The model under review builds one solid part; all positions refer to its coordinate system, in mm. A direction names the side the tool comes from. Give positions to 0.01 mm unless a question says otherwise; leave off trailing zeros. Order: outer loops, then holes, each group sorted by start corner. A loop starts at its lowest first (then second) coordinate and runs counter-clockwise, first axis right, second up. Notation, with made-up numbers: (35, 82.25) - (90, 82.25) arc R14 ccw to (90, 103.25) - close; hole circle Ø10 at (75.25, 77.5). An arc over 180 degrees is marked (long way). Write item = value, one per line. Start each with the question number.
1. For P1, Ø3, axis at y = 8, z = -2, coming from the -X side, flat-tipped, find the tip position at first contact; note if it passes through.
2. Machinability: for faces 4 (the flat face through (41, 5, 14.564)), 5 (the flat face through (-29.048, 8, 2)), which of the approach directions +Z, -Z, +X, -X, +Y, -Y give a long, thin tool a straight path to every point of the face, cutting with its end or side? Answer none if there is none.
3. We need section B-B, the plane z = 8.5. Give the boundary of the cut face in (x, y), and give its area (3 significant figures).
4. Wall thickness on probe 1 along X at (y, z) = (8.75, -5.5); probe 2 along Y at (x, z) = (-38.5, 4.75); probe 3 along X at (y, z) = (0.5, 8.5): over which ranges is each line inside the solid? List them lowest first.
5. We need section C-C, the plane z = -2.75. Give the boundary of the cut face in (x, y).
6. We need section A-A, the plane y = 3.5. Give the boundary of the cut face in (x, z).
7. Mouldability with a two-part tool opening along X and no side actions: class faces 1 (the cylindrical face through (-43.196, 2.958, 1.992)), 2 (the flat face through (47, 10, 2)), 3 (the cylindrical face through (-54.045, 2.958, 2.339)) as pulls with the +X half, pulls with the -X half, needs draft (parallel to the pull), parting line crosses it, or undercut.
from build123d import *

# Parameters (mm, degrees)
SKETCH1_R           = 1.65
BOSS_EXTRUDE1_DEPTH = 10
SKETCH2_W           = 29.50673097
SKETCH2_H           = 30.126833799
CUT_EXTRUDE1_DEPTH  = 4


with BuildPart() as part:
    # Sketch1 → Boss-Extrude1 (new body)
    with BuildSketch(Plane(origin=(0, 0, 0), x_dir=(1, 0, 0), z_dir=(0, 1, 0))):
        with BuildLine():
            Line((-41.547817516, 10.435693018), (120.952182484, 10.435693018))
            Line((120.952182484, 10.435693018), (120.952182484, -14.564306982))
            Line((120.952182484, -14.564306982), (-41.547817516, -14.564306982))
            ThreePointArc((-41.547817516, -14.564306982), (-54.047817516, -2.064306982), (-41.547817516, 10.435693018))
        make_face()
        with Locations((-41.547817516, -2.064306982)):
            Circle(SKETCH1_R, mode=Mode.SUBTRACT)
    extrude(amount=BOSS_EXTRUDE1_DEPTH)

    # Sketch2 → Cut-Extrude1 (cut)
    with BuildSketch(Plane(origin=(0, 10, 0), x_dir=(1, 0, 0), z_dir=(0, 1, 0))):
        with Locations((-43.801183001, 0.499109917)):
            Rectangle(SKETCH2_W, SKETCH2_H)
    extrude(amount=-CUT_EXTRUDE1_DEPTH, mode=Mode.SUBTRACT)


solid = part.part
Model answer:
q1.P1 = -29.05
q2.face_4 = +Z, +X, -X, +Y, -Y
q2.face_5 = +Z, -Z, -X, +Y
q3.outline = (-52.26, 0) - (120.95, 0) - (120.95, 10) - (-29.05, 10) - (-29.05, 6) - (-52.26, 6) - close
q3.area = 1,640 mm2
q4.probe_1 = -29.05 to 120.95
q4.probe_2 = 0 to 6
q4.probe_3 = -52.26 to 120.95
q5.outline = (-53.08, 0) - (120.95, 0) - (120.95, 10) - (-29.05, 10) - (-29.05, 6) - (-53.08, 6) - close
q6.outline = (-41.55, -10.44) - (120.95, -10.44) - (120.95, 14.56) - (-41.55, 14.56) arc R12.5 ccw to start; hole circle Ø3.3 at (-41.55, 2.06)
q7.face_1 = undercut
q7.face_2 = needs draft
q7.face_3 = pulls with the -X half
